Autodesk Inventor part; units mm, degrees
ref_plane "YZ Plane" through (0, 0, 0) normal (1, 0, 0) x (0, 1, 0)
ref_plane "XZ Plane" through (0, 0, 0) normal (0, 1, 0) x (-1, 0, 0)
ref_plane "XY Plane" through (0, 0, 0) normal (0, 0, 1) x (1, 0, 0)
sketch "草圖1" plane through (0, 0, 0) normal (0, 0, 1) x (1, 0, 0)
  circle A0 centre (0, 0) radius 10
  arc A1 (20, 0) -> (-20, 0) centre (0, 0) ccw
  line L0 (-20, 0) -> (-20, -20)
  line L1 (-20, -20) -> (40, -20)
  line L2 (40, -20) -> (40, -10)
  line L3 (40, -10) -> (-20, -10)
  line L4 (-20, -10) -> (-20, -20)
  line L5 (20, 0) -> (30, 0)
  line L6 (40, -10) -> (40, -10)
  arc A2 (40, -10) -> (30, 0) centre (30, -10) ccw
  point P0 (40, 0)
  point P1 (0, -10)
extrude "擠出1" add sketch "草圖1" along normal blind 30 contours L3 L2 L1 L0
extrude "擠出2" add sketch "草圖1" along normal blind 20 contours L3 L0 A1 L5 A2
CAD build for the part. Positions are in the model's coordinates, mm. A direction names the side the tool comes from. Coordinates: 2 decimals unless noted, no trailing zeros. Write each loop counter-clockwise with the first axis right and the second up, starting at its lowest first coordinate (ties: lowest second). Pieces come first, ordered by that corner, then holes. Notation, with made-up numbers: M -19.5,40.5 L 28.5,40.5 A24 cw 28.5,50.5 Z; hole C -21,44.25 d4. An arc over 180 degrees is marked long. Answer as a JSON object with one key per item and string values. Group by question number.
1) Saw through at C-C (x = 21). Write the cut outline in (y, z).
2) Wall check: line 1 (Y direction, x = 0, z = 6); line 2 (Y direction, x = 28.5, z = 6.75); line 3 (Z direction, x = 23.5, y = -2). Give the ranges that are in metal, low to high. Write a range as from..to.
3) Saw through at A-A (y = 3). Write the cut outline in (x, z).
4) Tool access for faces 1 (the face through (25, 0, 10)), 2 (the face through (10, -10, 25)), 3 (the face through (40, -15, 15)): list every direction of +Z, -Z, +X, -X, +Y, -Y with a clear straight run to the whole face (end or side of a thin tool).
5) Saw through at D-D (y = 8). Write the cut outline in (x, z), plus the area to 3 significant figures.
6) Saw through at B-B (z = 9.75). Write the cut outline in (x, y).
7) Mould opens along Y. For faces 4 (the face through (10, 5, 20)), 5 (the face through (36.99, -2.85, 9.86)), 6 (the face through (-2.17, 9.76, 9.86)) say: +Y half, -Y half, draft (parallel to the pull), parting line (faces both ways), or undercut.
8) Pin check, flat tips, straight feed: pin 1 Ø10 at (x, y) = (17.5, 8) entering from +Z; pin 2 Ø10 at (x, z) = (21.5, 25.5) entering from +Y; pin 3 Ø3 at (x, z) = (27.5, 10.5) entering from +Y. Stop position of each tip, or through.
Values follow:
{
 "1": {"outline": "M -20,0 L 0,0 L 0,20 L -10,20 L -10,30 L -20,30 Z"},
 "2": {"line 1": "y = -20..-10, 10..20", "line 2": "y = -20..0", "line 3": "z = 0..20"},
 "3": {"outline": "M -19.77,0 L -9.54,0 L -9.54,20 L -19.77,20 Z; M 9.54,0 L 19.77,0 L 19.77,20 L 9.54,20 Z"},
 "4": {"face 1": "+Z, -Z, +X, +Y", "face 2": "+Z, +X, -X, +Y", "face 3": "+Z, -Z, +X, +Y, -Y"},
 "5": {"outline": "M -18.33,0 L -6,0 L -6,20 L -18.33,20 Z; M 6,0 L 18.33,0 L 18.33,20 L 6,20 Z", "area": "493 mm2"},
 "6": {"outline": "M -20,-20 L 40,-20 L 40,-10 A10 ccw 30,0 L 20,0 A20 ccw -20,0 Z; hole C 0,0 d20"},
 "7": {"face 4": "draft", "face 5": "+Y half", "face 6": "undercut"},
 "8": {"pin 1": "stops at z = 20", "pin 2": "stops at y = -10", "pin 3": "stops at y = 0"}
}
